Geometry: final body of the model. Coordinates: model frame, mm. A direction names the side the tool comes from. Coordinates: 2 decimals unless noted, no trailing zeros. Write each loop counter-clockwise with the first axis right and the second up, starting at its lowest first coordinate (ties: lowest second). Pieces come first, ordered by that corner, then holes.
from build123d import *

# Parameters (mm, degrees)
SKETCH1_W                        = 20
SKETCH1_H                        = 10
BOSS_EXTRUDE1_DEPTH              = 5
BOSS_EXTRUDE2_DEPTH              = 20
CUT_EXTRUDE1_DEPTH               = 4.09576
FILLET1_R                        = 0.5
CUT_EXTRUDE2_REACH               = 35.208
CUT_EXTRUDE2_OFFSET_FROM_SURFACE = 1
SKETCH4_R                        = 0.5


with BuildPart() as part:
    # Sketch1 → Boss-Extrude1 (new body)
    with BuildSketch(Plane.XY):
        with Locations((-83, 16.5)):
            Rectangle(SKETCH1_W, SKETCH1_H)
    extrude(amount=BOSS_EXTRUDE1_DEPTH)

    # Sketch2 → Boss-Extrude2 (add)
    with BuildSketch(Plane.ZY.offset(93)):
        Polygon((5, 16.5), (1.498962309, 11.5), (6.498962309, 11.5), (32.208054955, 48.216389418), (32.208054955, 55.357129452), (8.501037691, 21.5), (5, 21.5), align=None)
    extrude(amount=-BOSS_EXTRUDE2_DEPTH)

    # Sketch3 → Cut-Extrude1 (cut)
    with BuildSketch(Plane(origin=(0, 3.079102266, -4.397413763), x_dir=(-1, 0, 0), z_dir=(0, 0.573576436, -0.819152044))):
        Polygon((90.5, 29.170685305), (90.5, 36.425657649), (86.606804382, 33.925761075), align=None)
        Polygon((76.580636571, 27.487763856), (89.293048323, 27.487763856), (84.912643674, 32.837907557), align=None)
        Polygon((79.020661139, 31.431370249), (75.5, 42.221469006), (75.5, 29.170685305), align=None)
        Polygon((83.682826439, 48.850072065), (75.5, 50.589500561), (75.5, 48.669091242), (77.437703633, 42.730430083), align=None)
        Polygon((77.812370658, 52.142645531), (81.816362113, 58.81968714), (75.5, 58.81968714), (75.5, 52.634187597), align=None)
        Polygon((90.5, 55.53027081), (90.5, 58.81968714), (84.148398738, 58.81968714), (83.395113947, 57.563512158), (88.334689519, 53.40846707), align=None)
        Polygon((86.899562452, 52.002175453), (85.397480311, 50.530274064), (79.880748536, 51.702969161), (82.353375162, 55.826312344), align=None)
        Polygon((90.5, 38.802476843), (90.5, 52.730114749), (88.38308654, 50.655735608), (88.38308654, 37.443165566), align=None)
        Polygon((86.38308654, 36.158926695), (80.76001209, 32.548241301), (78.130006045, 40.608666271), (86.38308654, 48.69592083), align=None)
    extrude(amount=-CUT_EXTRUDE1_DEPTH, mode=Mode.SUBTRACT)

    # Fillet1
    fillet1_edges = [part.edges().sort_by_distance(p)[0] for p in [
        (-88.38308654, 39.162299764, 20.868313128),
        (-90.5, 40.568657026, 21.853055085),
        (-89.44154327, 34.307489189, 17.468938167),
        (-89.44154327, 45.423467601, 25.252430045),
        (-85.864901733, 48.530564087, 27.428042427),
        (-90.5, 49.914103175, 28.396806926),
        (-87.324199369, 51.26136923, 29.340172774),
        (-89.41734476, 47.697797184, 26.844932764),
        (-83.771756342, 50.746870078, 28.979916589),
        (-84.626468807, 47.243065371, 26.526526121),
        (-81.117061849, 47.120517648, 26.440717281),
        (-82.639114423, 44.951387357, 24.9218759),
        (-86.148521381, 45.07393508, 25.007684739),
        (-88.553402191, 31.893356499, 15.778544259),
        (-88.553402191, 28.921893785, 13.697903667),
        (-90.5, 29.94579148, 14.414844551),
        (-83, 21.5, 8.501037691),
        (-83, 55.357129452, 32.208054955),
        (-83, 11.5, 6.498962309),
        (-93, 29.858194709, 19.353508632),
        (-93, 38.428564726, 20.354546323),
        (-73, 38.428564726, 20.354546323),
        (-73, 29.858194709, 19.353508632),
        (-80.560265036, 40.588280041, 21.866795268),
        (-76.468851816, 40.514154635, 21.814892099),
        (-79.59141322, 43.807166866, 24.120684086),
        (-75.5, 43.73304146, 24.068780918),
        (-73, 11.5, 3.249481154),
        (-76.656185329, 45.993180791, 25.651347516),
        (-93, 11.5, 3.249481154),
        (-79.814366386, 48.526613089, 27.425275908),
        (-78.658181056, 51.26136923, 29.340172774),
        (-75.5, 48.727936933, 27.566244381),
        (-93, 21.5, 4.250518846),
        (-73, 21.5, 4.250518846),
        (-87.102845999, 27.787050796, 12.903278052),
        (-80.746640123, 27.787050796, 12.903278052),
        (-82.936842447, 25.595760221, 11.368919873),
        (-77.26033057, 27.900251113, 12.982541767),
        (-77.26033057, 33.245539188, 16.725352771),
        (-75.5, 32.319616841, 16.077014963),
        (-86.38308654, 37.833613175, 19.937956762),
        (-82.256546293, 39.65611981, 21.214089647),
        (-79.445009068, 33.042417461, 16.583125407),
        (-83.571549315, 31.219910826, 15.306992522),
    ]]
    fillet(fillet1_edges, radius=FILLET1_R)

    # Cut-Extrude2: up to this face of the body (flat: up to its plane, moved by the offset)
    cut_extrude2_end = Plane(part.part.faces().sort_by_distance((-83.030327421, 27.270141069, 17.541333964))[0]).offset(-CUT_EXTRUDE2_OFFSET_FROM_SURFACE)
    # Sketch4 → Cut-Extrude2 (cut, up to the picked face)
    with BuildSketch(Plane(origin=(0, 0, 0), x_dir=(-1, 0, 0), z_dir=(0, 0, -1)), mode=Mode.PRIVATE) as cut_extrude2_sk1:
        with Locations((78, 16.5)):
            Circle(SKETCH4_R)
    cut_extrude2_tool1 = split(extrude(cut_extrude2_sk1.sketch, amount=-CUT_EXTRUDE2_REACH, mode=Mode.PRIVATE), bisect_by=cut_extrude2_end, keep=Keep.BOTH, mode=Mode.PRIVATE)
    add(cut_extrude2_tool1.solids().sort_by_distance((-78, 16.5, 0))[0], mode=Mode.SUBTRACT)
    # Sketch4 → Cut-Extrude2 (cut, up to the picked face)
    with BuildSketch(Plane(origin=(0, 0, 0), x_dir=(-1, 0, 0), z_dir=(0, 0, -1)), mode=Mode.PRIVATE) as cut_extrude2_sk2:
        with Locations((88, 16.5)):
            Circle(SKETCH4_R)
    cut_extrude2_tool2 = split(extrude(cut_extrude2_sk2.sketch, amount=-CUT_EXTRUDE2_REACH, mode=Mode.PRIVATE), bisect_by=cut_extrude2_end, keep=Keep.BOTH, mode=Mode.PRIVATE)
    add(cut_extrude2_tool2.solids().sort_by_distance((-88, 16.5, 0))[0], mode=Mode.SUBTRACT)


solid = part.part
Item 1: Pin query (flat end, axial travel): pin 1 (9 mm diameter, centred on x = -87.5, z = 4, fed in from +Y); pin 2 (12 mm diameter, centred on x = -89, z = 9, fed in from +Y); pin 3 (3 mm diameter, centred on x = -79, y = 35.5, fed in from -Z). Return the tip coordinate at first contact, or that it passes through.
Derived:
pin 1: stops at y = 21.57
pin 2: stops at y = 30.32
pin 3: stops at z = 17.3
Item 2: Section B-B, the plane x = -91.5. Output: boundary loops of the cut face in (y, z), plus the area to 3 significant figures.
Derived:
outline: (11.5, 0) - (21.5, 0) - (21.5, 8.24) arc R0.5 cw to (21.71, 8.65) - (54.06, 31.3) arc R0.5 ccw to (53.77, 32.21) - (48.22, 32.21) - (11.71, 6.65) arc R0.5 ccw to (11.5, 6.24) - close
area: 251 mm2
Item 3: Material intervals for probe 1 along X at (y, z) = (16.5, 4.25); probe 2 along Y at (x, z) = (-78, 6); probe 3 along Z at (x, y) = (-87.25, 29), sorted ascending.
Derived:
probe 1: x = -93 to -88.5, -87.5 to -78.5, -77.5 to -73
probe 2: y = 11.5 to 16, 17 to 21.5
probe 3: z = 13.75 to 16.36, 18.45 to 18.75
Item 4: Pull-direction query (X, two-part tool) for faces 6 (the flat face through (-79.786, 47.185, 29.26)), 7 (the flat face through (-73, 27, 14)), 8 (the flat face through (-88.526, 27.646, 15.579)), 9 (the cylindrical face through (-92.86, 37.77, 20.08)); classes: released by +X, released by -X, zero draft, split by the parting line, or undercut.
Derived:
face 6: undercut
face 7: released by +X
face 8: undercut
face 9: released by -X
Item 5: Set-up query: faces 1 (the flat face through (-83.61, 29.94, 17.18)), 2 (the flat face through (-89.4, 46.38, 28.7)), 3 (the cylindrical face through (-73.15, 37.779, 20.074)), 4 (the cylindrical face through (-89.27, 33.99, 17.42)), 5 (the cylindrical face through (-77.456, 33.069, 16.776)). Return all of +Z, -Z, +X, -X, +Y, -Y with unobstructed straight access to the full face (end or side cutting, diameter ignored); none if empty.
Derived:
face 1: +Z, +Y
face 2: +Z
face 3: -Z, +X, +Y
face 4: +Y
face 5: -Z
Item 6: Section C-C, the plane y = 39. State how many separate pieces and enclosed holes the cut face has, plus the area to 3 significant figures.
Derived:
separate pieces: 4
enclosed holes: 0
area: 54.1 mm2
Item 7: Section A-A, the plane z = 3. Output: boundary loops of the cut face in (x, y), plus the area to 3 significant figures.
Derived:
outline: (-93, 12) arc R0.5 ccw to (-92.5, 11.5) - (-73.5, 11.5) arc R0.5 ccw to (-73, 12) - (-73, 21) arc R0.5 ccw to (-73.5, 21.5) - (-92.5, 21.5) arc R0.5 ccw to (-93, 21) - close; hole circle Ø1 at (-88, 16.5); hole circle Ø1 at (-78, 16.5)
area: 198 mm2
